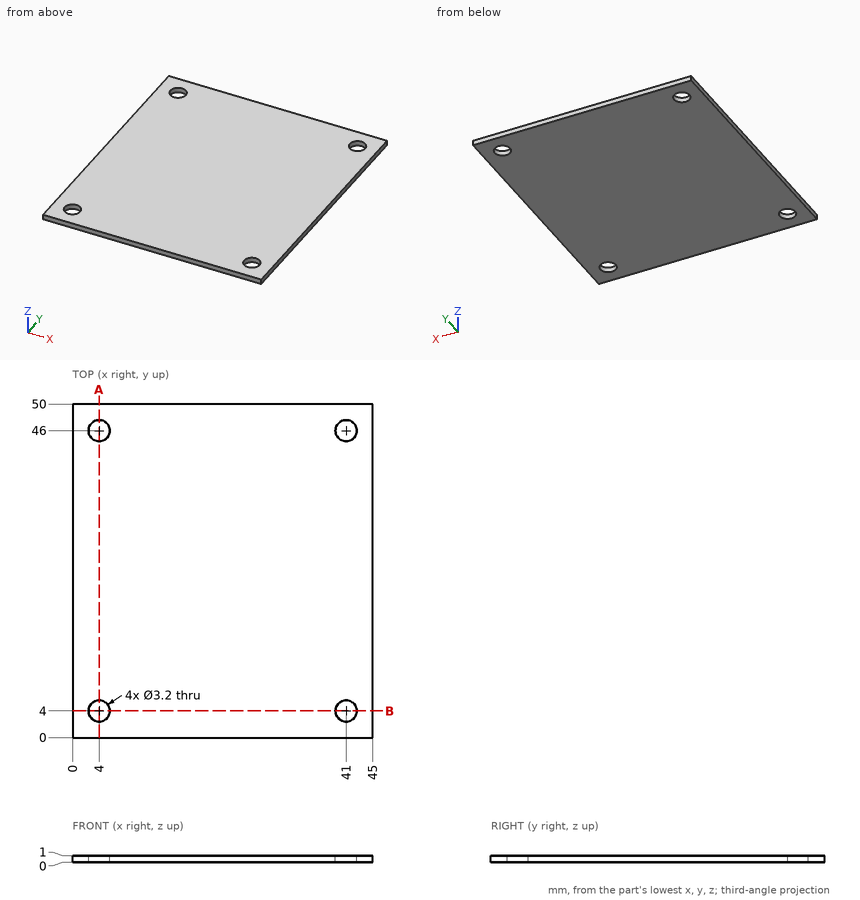
Design review of the part shown in the three views and the two pictorial views. Dimensions are in mm from the part's minimum x, y and z. Give positions to 0.01 mm unless a question says otherwise; leave off trailing zeros. Loops run counter-clockwise (first coordinate to the right, second up) from the corner with the lowest first, then second, coordinate; pieces in that order, holes last. Notation, with made-up numbers: M 65,0 L 116,0 A30 ccw 116,29 Z; hole C 66,38.25 d5. An arc over 180 degrees is marked long. Answer as a JSON object with one key per item and string values. Group by question number.
Q1. Add section B-B on y = 4. Give the boundary of the cut face in (x, z).
Q2. Add section A-A on x = 4. Give the boundary of the cut face in (y, z).
Q3. For probe 1 along X at (y, z) = (4, 0.55); probe 2 along Y at (x, z) = (4, 0.7); probe 3 along X at (y, z) = (47, 0.8), list the stretches that pass through material, from the lowest coordinate up. Write a range as [from, to].
Q4. Insertion check: P1, Ø2.5, axis at x = 41, y = 46, coming from the +Z side. The pin has a flat end and moves straight along its axis. Give the tip position at first contact, or say it passes through.
Checked values:
{
 "1": {"outline": "M 0,0 L 2.4,0 L 2.4,1 L 0,1 Z; M 5.6,0 L 39.4,0 L 39.4,1 L 5.6,1 Z; M 42.6,0 L 45,0 L 45,1 L 42.6,1 Z"},
 "2": {"outline": "M 0,0 L 2.4,0 L 2.4,1 L 0,1 Z; M 5.6,0 L 44.4,0 L 44.4,1 L 5.6,1 Z; M 47.6,0 L 50,0 L 50,1 L 47.6,1 Z"},
 "3": {"probe 1": "[0, 2.4], [5.6, 39.4], [42.6, 45]", "probe 2": "[0, 2.4], [5.6, 44.4], [47.6, 50]", "probe 3": "[0, 2.75], [5.25, 39.75], [42.25, 45]"},
 "4": {"P1": "through"}
}
